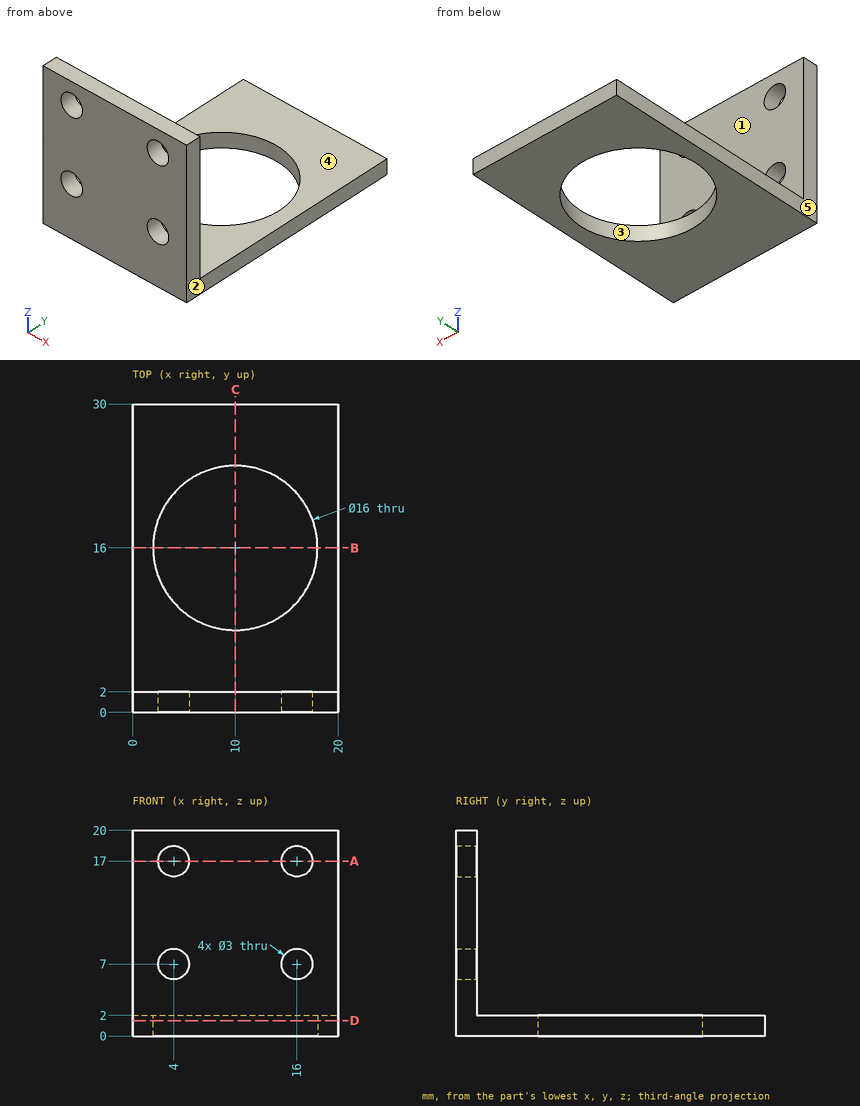
For this review, use the dimensioned drawing (mm, ordinates from the lowest corner) and the shaded views. A direction names the side the tool comes from. Round coordinates to 2 decimals unless told otherwise and drop trailing zeros. Write each loop counter-clockwise with the first axis right and the second up, starting at its lowest first coordinate (ties: lowest second). Pieces come first, ordered by that corner, then holes. Notation, with made-up numbers: M -7.5,25 L 23.5,25 A36 cw 23.5,62 Z; hole C 1,-12 d11. An arc over 180 degrees is marked long. Use CSV: the item, a comma, the result in double quotes. Start each with the question number.
(1) We need section B-B, the plane y = 16. State the section outline as (x, z) points, then the cut area to 3 significant figures.
(2) Tool access review of the marked faces 4 and 5: name each direction out of +Z, -Z, +X, -X, +Y, -Y from which nothing blocks a thin tool from reaching the whole face with its end or side.
(3) The part is to be moulded in two halves that separate along X. For the marked faces 1, 2 and 3, say which applies: +X half, -X half, draft (parallel to the pull), parting line (faces both ways), or undercut.
(4) We need section D-D, the plane z = 1.5. State the section outline as (x, y) points, then the cut area to 3 significant figures.
(5) We need section A-A, the plane z = 17. State the section outline as (x, y) points, then the cut area to 3 significant figures.
(6) We need section C-C, the plane x = 10. State the section outline as (y, z) points.
(7) Clearance check with flat-ended pins moving along their axes: P1, Ø4, axis at x = 4, z = 7, coming from the +Y side; P2, Ø3, axis at x = 16.5, y = 17.5, coming from the +Z side; P3, Ø1.8, axis at x = 16, z = 7, coming from the +Y side. State where each tip first meets the part, or that it passes through.
(8) For line 1 along Z through (x, y) = (16, 0.55); line 2 along X through (y, z) = (1.1, 7); line 3 along Y through (x, z) = (10, 0.7), list the stretches that pass through material, from the lowest coordinate up.
Findings:
1,outline,"M 0,0 L 2,0 L 2,2 L 0,2 Z; M 18,0 L 20,0 L 20,2 L 18,2 Z"
1,area,"8.00 mm^2"
2,face 4,"+Z, +X, -X, +Y"
2,face 5,"+Z, -Z, -X, +Y, -Y"
3,face 1,"draft"
3,face 2,"+X half"
3,face 3,"undercut"
4,outline,"M 0,0 L 20,0 L 20,30 L 0,30 Z; hole C 10,16 d16"
4,area,"399 mm^2"
5,outline,"M 0,0 L 2.5,0 L 2.5,2 L 0,2 Z; M 5.5,0 L 14.5,0 L 14.5,2 L 5.5,2 Z; M 17.5,0 L 20,0 L 20,2 L 17.5,2 Z"
5,area,"28.0 mm^2"
6,outline,"M 0,0 L 8,0 L 8,2 L 2,2 L 2,20 L 0,20 Z; M 24,0 L 30,0 L 30,2 L 24,2 Z"
7,P1,"y = 2"
7,P2,"z = 2"
7,P3,"through"
8,line 1,"0 to 5.5, 8.5 to 15.5, 18.5 to 20"
8,line 2,"0 to 2.5, 5.5 to 14.5, 17.5 to 20"
8,line 3,"0 to 8, 24 to 30"
